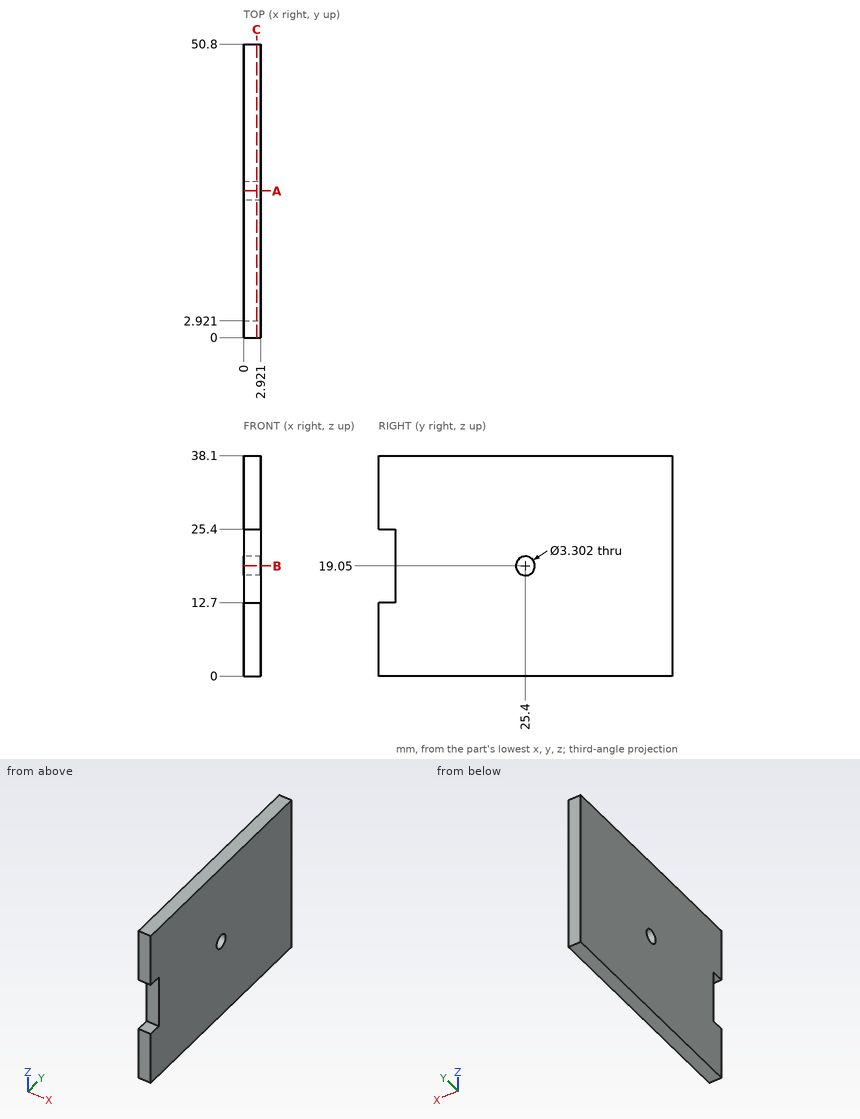
Job drawing, mm, ordinate dimensions from the low corner. One solid piece. Coordinates: 2 decimals unless noted, no trailing zeros. Order: outer loops, then holes, each group sorted by start corner. A loop starts at its lowest first (then second) coordinate and runs counter-clockwise, first axis right, second up. Notation, with made-up numbers: (21.5, 73) -> (63.5, 73) arc R24 ccw to (63.5, 112) -> close; hole circle Ø9 at (81, 8). An arc over 180 degrees is marked (long way). Answer in a Markdown table with one row per item. Add a question column.
Q1. Band-saw the part on B-B, the plane z = 19.05. List the corners of the cut face in (x, y).
Q2. Band-saw the part on C-C, the plane x = 2.25. List the corners of the cut face in (y, z).
Q3. Band-saw the part on A-A, the plane y = 25.4. List the corners of the cut face in (x, z), then the cut area to 3 significant figures.
Q4. Wall check: line 1 along Z through (x, y) = (1.7, 25.4); line 2 along Y through (x, z) = (1.35, 16.5); line 3 along Z through (x, y) = (0.95, 26). Give the ranges that are in metal, low to high. Write a range as [from, to].
Answers follow:
| question | item | result |
|---|---|---|
| 1 | outline | (0, 2.92) -> (2.92, 2.92) -> (2.92, 23.75) -> (0, 23.75) -> close; (0, 27.05) -> (2.92, 27.05) -> (2.92, 50.8) -> (0, 50.8) -> close |
| 2 | outline | (0, 0) -> (50.8, 0) -> (50.8, 38.1) -> (0, 38.1) -> (0, 25.4) -> (2.92, 25.4) -> (2.92, 12.7) -> (0, 12.7) -> close; hole circle Ø3.3 at (25.4, 19.05) |
| 3 | outline | (0, 0) -> (2.92, 0) -> (2.92, 17.4) -> (0, 17.4) -> close; (0, 20.7) -> (2.92, 20.7) -> (2.92, 38.1) -> (0, 38.1) -> close |
| 3 | area | 102 mm^2 |
| 4 | line 1 | [0, 17.4], [20.7, 38.1] |
| 4 | line 2 | [2.92, 50.8] |
| 4 | line 3 | [0, 17.51], [20.59, 38.1] |
